```python
from build123d import *

# Parameters (mm, degrees)
F1_DEPTH = 350
F3_DEPTH = 20
F5_D     = 5


with BuildPart() as f1:
    # F0 (on Front) → F1 (new body)
    with BuildSketch(Plane.XZ):
        with BuildLine():
            Line((-9.55, 2.17), (-9.55, 0))
            Line((-9.55, 0), (9.55, 0))
            Line((9.55, 0), (9.55, 2.17))
            ThreePointArc((9.55, 2.17), (9.257107, 2.877107), (8.55, 3.17))
            Line((8.55, 3.17), (2.585, 3.17))
            ThreePointArc((2.585, 3.17), (1.877893, 3.462893), (1.585, 4.17))
            Line((1.585, 4.17), (1.585, 18.1))
            ThreePointArc((1.585, 18.1), (1.292107, 18.807107), (0.585, 19.1))
            Line((0.585, 19.1), (-0.585, 19.1))
            ThreePointArc((-0.585, 19.1), (-1.292107, 18.807107), (-1.585, 18.1))
            Line((-1.585, 18.1), (-1.585, 4.17))
            ThreePointArc((-1.585, 4.17), (-1.877893, 3.462893), (-2.585, 3.17))
            Line((-2.585, 3.17), (-8.55, 3.17))
            ThreePointArc((-8.55, 3.17), (-9.257107, 2.877107), (-9.55, 2.17))
        make_face()
    extrude(amount=F1_DEPTH)

    # F2 (on face) → F3 (cut)
    with BuildSketch(Plane(origin=(0, 0, 0), x_dir=(1, 0, 0), z_dir=(0, 0, -1))):
        Polygon((-9.55, 330.9), (9.55, 350), (-9.55, 350), align=None)
        Polygon((-9.55, 0), (9.55, 0), (-9.55, 19.1), align=None)
    extrude(amount=-F3_DEPTH, mode=Mode.SUBTRACT)

    # F5 (through all)
    with Locations(Plane(origin=(0, 0, 0), x_dir=(1, 0, 0), z_dir=(0, 0, -1))):
        with Locations((5.55, 310), (5.55, 40)):
            Hole(F5_D / 2)


solid = f1.part
```
Build history of the part. All positions in model axes, mm. A direction names the side the tool comes from. Give positions to 0.01 mm unless a question says otherwise; leave off trailing zeros. Order: outer loops, then holes, each group sorted by start corner. A loop starts at its lowest first (then second) coordinate and runs counter-clockwise, first axis right, second up. Notation, with made-up numbers: M -15.5,55.25 L 5.5,55.25 A26 cw 5.5,74.25 Z; hole C 1.5,70 d9. An arc over 180 degrees is marked long. Write item = value, one per line. Start each with the question number.
(1) Probe L1, parallel to X at y = -310, z = 1; L2, parallel to Y at x = 5.55, z = 1.9. List the from-to ranges inside material, lowest first. Write a range as [from, to].
(2) Pin check, flat tips, straight feed: pin 1 Ø6.5 at (x, y) = (-5.5, -188.5) entering from +Z; pin 2 Ø2 at (x, z) = (6, 3.5) entering from +Y; pin 3 Ø10 at (x, z) = (5, 16) entering from -Y (3 decimals); pin 4 Ø6 at (x, y) = (-0.5, -120.5) entering from -Z. Stop position of each tip, or through.
(3) Which spindle directions (+Z, -Z, +X, -X, +Y, -Y) get a long thin tool onto all of the face, cutting with end or side? Do faces 1 (the flat face through (-6, -173, 3.17)), 2 (the flat face through (6, -173, 3.17)), 3 (the flat face through (0, -173, 0)). Say none if no direction does.
(4) Slice it at B-B on z = 11. Write the cut outline in (x, y) (3 decimals), plus the area to 3 significant figures.
(5) Slice it at A-A on y = -108.5. Write the cut outline in (x, z) (3 decimals).
Responses:
q1.L1 = [-9.55, 3.05], [8.05, 9.55]
q1.L2 = [-346, -312.5], [-307.5, -42.5], [-37.5, -4]
q2.pin_1 = 3.23
q2.pin_2 = -2.61
q2.pin_3 = -342.035
q2.pin_4 = 0
q3.face_1 = +Z, -X, +Y, -Y
q3.face_2 = +Z, +X, +Y, -Y
q3.face_3 = -Z, +X, -X, +Y, -Y
q4.outline = M -1.585,-338.865 L 1.585,-342.035 L 1.585,-7.965 L -1.585,-11.135 Z
q4.area = 1,050 mm2
q5.outline = M -9.55,0 L 9.55,0 L 9.55,2.17 A1 ccw 8.55,3.17 L 2.585,3.17 A1 cw 1.585,4.17 L 1.585,18.1 A1 ccw 0.585,19.1 L -0.585,19.1 A1 ccw -1.585,18.1 L -1.585,4.17 A1 cw -2.585,3.17 L -8.55,3.17 A1 ccw -9.55,2.17 Z
